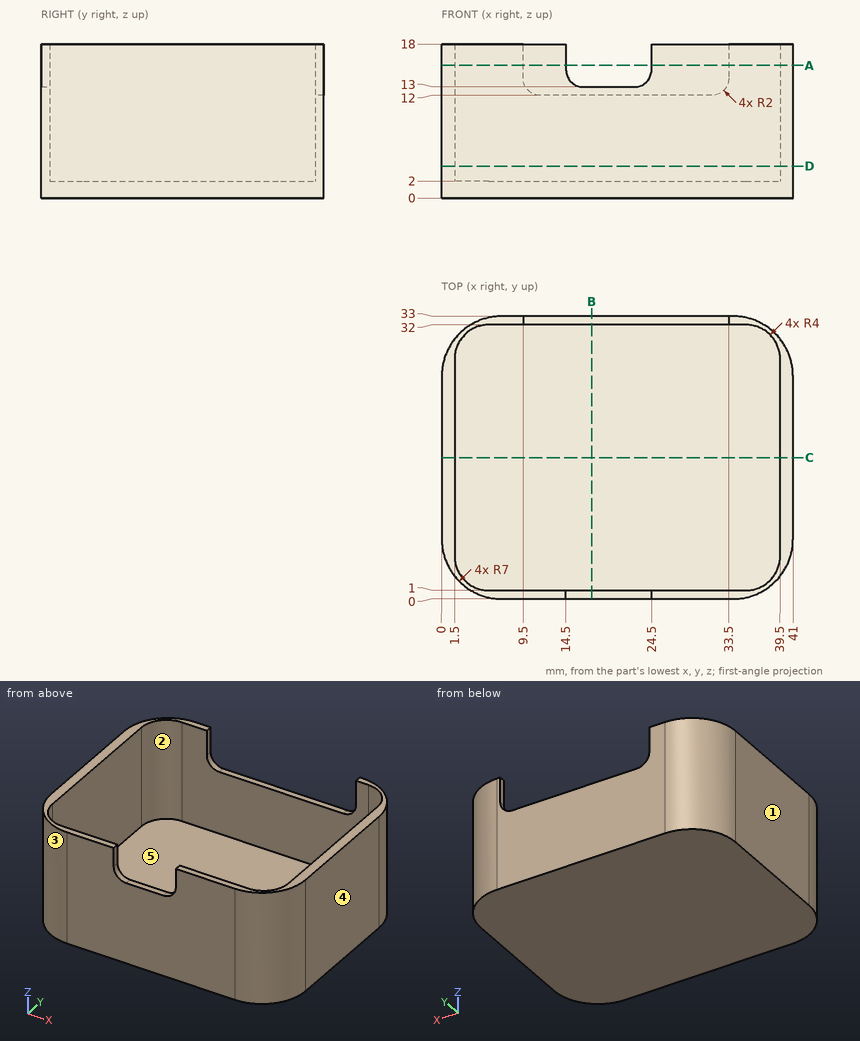
Part print with two shaded views. Sizes in mm from the minimum x, y, z corner. A direction names the side the tool comes from. Give positions to 0.01 mm unless a question says otherwise; leave off trailing zeros. Order: outer loops, then holes, each group sorted by start corner. A loop starts at its lowest first (then second) coordinate and runs counter-clockwise, first axis right, second up.
1) Saw through at D-D, the plane z = 3.75. Write the cut outline in (x, y).
2) Mould opens along Y. For the marked faces 3, 4 and 5 say: +Y half, -Y half, draft (parallel to the pull), parting line (faces both ways), or undercut.
3) Wall check: probe 1 along Y at (x, z) = (8, 3.5); probe 2 along X at (y, z) = (13, 2.75); probe 3 along Z at (x, y) = (18, 8.5). Give the ranges that are in metal, low to high.
4) Saw through at B-B, the plane x = 17.5. Write the cut outline in (y, z).
5) Saw through at C-C, the plane y = 16.5. Write the cut outline in (x, z), then the cut area to 3 significant figures.
6) Saw through at A-A, the plane z = 15.5. Write the cut outline in (x, y).
7) Pin check, flat tips, straight feed: pin 1 (1.1 mm diameter, centred on y = 0.5, z = 16.5, fed in from +X); pin 2 (0.5 mm diameter, centred on y = 32.5, z = 17, fed in from +X); pin 3 (3 mm diameter, centred on x = 20.5, y = 9.5, fed in from -Z); pin 4 (1.1 mm diameter, centred on x = 20, y = 0.5, fed in from +Z). Stop position of each tip, or through.
8) 3-axis set-ups, long thin cutter, end or side, ignore diameter. For the marked faces 1 and 2: which of +Z, -Z, +X, -X, +Y, -Y reach the whole face in a straight line?
Computed:
1. outline: (0, 7) arc R7 ccw to (7, 0) - (34, 0) arc R7 ccw to (41, 7) - (41, 26) arc R7 ccw to (34, 33) - (7, 33) arc R7 ccw to (0, 26) - close; hole (1.5, 5) arc R4 ccw to (5.5, 1) - (35.5, 1) arc R4 ccw to (39.5, 5) - (39.5, 28) arc R4 ccw to (35.5, 32) - (5.5, 32) arc R4 ccw to (1.5, 28) - close
2. face 3: -Y half
2. face 4: draft
2. face 5: undercut
3. probe 1: y = 0 to 1, 32 to 33
3. probe 2: x = 0 to 1.5, 39.5 to 41
3. probe 3: z = 0 to 2
4. outline: (0, 0) - (33, 0) - (33, 12) - (32, 12) - (32, 2) - (1, 2) - (1, 13) - (0, 13) - close
5. outline: (0, 0) - (41, 0) - (41, 18) - (39.5, 18) - (39.5, 2) - (1.5, 2) - (1.5, 18) - (0, 18) - close
5. area: 130 mm2
6. outline: (0, 7) arc R7 ccw to (7, 0) - (14.5, 0) - (14.5, 1) - (5.5, 1) arc R4 cw to (1.5, 5) - (1.5, 28) arc R4 cw to (5.5, 32) - (9.5, 32) - (9.5, 33) - (7, 33) arc R7 ccw to (0, 26) - close; (24.5, 0) - (34, 0) arc R7 ccw to (41, 7) - (41, 26) arc R7 ccw to (34, 33) - (33.5, 33) - (33.5, 32) - (35.5, 32) arc R4 cw to (39.5, 28) - (39.5, 5) arc R4 cw to (35.5, 1) - (24.5, 1) - close
7. pin 1: stops at x = 37.69
7. pin 2: stops at x = 37.15
7. pin 3: stops at z = 0
7. pin 4: stops at z = 13
8. face 1: +Z, -Z, -X, +Y, -Y
8. face 2: +Z
